from build123d import *

# Parameters (mm, degrees)
REVOLVE1_ANGLE = 180


with BuildPart() as part:
    # Sketch4 → Revolve1 (revolve)
    with BuildSketch(Plane(origin=(0, 0, 0), x_dir=(0, 0, -1), z_dir=(1, 0, 0))):
        with BuildLine():
            Line((0, 43.554228777), (0, 0))
            Line((0, 0), (-19.05, 0))
            Line((-19.05, 0), (-19.05, 10.16))
            Line((-19.05, 10.16), (-21.1117011, 10.795))
            Line((-21.1117011, 10.795), (-22.767765969, 12.084590197))
            Line((-22.767765969, 12.084590197), (-22.767765969, 13.323327865))
            Line((-22.767765969, 13.323327865), (-21.1117011, 14.680643181))
            Line((-21.1117011, 14.680643181), (-19.05, 15.24))
            add(Edge.make_bspline(
                [(-19.05, 15.24), (-24.619555557, 24.713120096), (-15.24, 32.969594186)],
                knots=[0, 0, 0, 1, 1, 1], degree=2))
            add(Edge.make_bspline(
                [(-15.24, 32.969594186), (-13.159056011, 34.466761199), (-10.754138268, 36.044746883), (-8.242416232, 37.433272674), (-7.973778325, 37.578839171)],
                knots=[0, 0, 0, 0, 0.730138174, 0.817134496, 0.817134496, 0.817134496, 0.817134496], degree=3))
            ThreePointArc((-7.973778325, 37.578839171), (-6.612881823, 38.215201507), (-5.186361227, 38.686407728))
            add(Edge.make_bspline(
                [(-5.186361227, 38.686407728), (-3.351057226, 39.150966228), (-2.104803263, 40.656792731), (-1.118621699, 42.156292635)],
                knots=[0, 0, 0, 0, 1, 1, 1, 1], degree=3))
            add(Edge.make_bspline(
                [(-1.118621699, 42.156292635), (-0.886078473, 43.158491049), (0, 43.554228777)],
                knots=[0, 0, 0, 1, 1, 1], degree=2))
        make_face()
    revolve(axis=Axis((0, 43.554228777, 0), (0, -1, 0)), revolution_arc=REVOLVE1_ANGLE)


solid = part.part
Input: part model. Units: mm. Frame: model coordinates. Coordinates: 2 decimals unless noted, no trailing zeros. Write item = value, one per line. Start each with the question number.
(1) First-contact query: P1, Ø5, axis at x = -7, z = 11, coming from the +Y side; P2, Ø6, axis at y = 30.5, z = 4, coming from the -X side; P3, Ø4, axis at x = -18, y = 24.5, coming from the +Z side. Flat tips, straight axial feed; report the tip coordinate or a pass-through.
(2) Line query: line 1 along Y through (x, z) = (-16, -11); line 2 along Y through (x, z) = (-16, -1.5); line 3 along Y through (x, z) = (-8.5, 9.5). Output: solid intervals per line, ascending. Write a range as [from, to].
(3) Pull-direction query (Y, two-part tool) for faces 1 (the cylindrical face through (-19.045, 5.151, 0.419)), 2 (the flat face through (-8, 0, 0)), 3 (the conical face through (-19.37, 15.15, 0.43)); classes: released by +Y, released by -Y, zero draft, split by the parting line, or undercut.
Result set:
q1.P1 = 36.1
q1.P2 = -19.43
q1.P3 = 13.47
q2.line_1 = [10.27, 15.14], [15.89, 28.09]
q2.line_2 = [0, 32.21]
q2.line_3 = [0, 34.69]
q3.face_1 = zero draft
q3.face_2 = released by -Y
q3.face_3 = undercut
